```python
from build123d import *

# Parameters (mm, degrees)
SKETCH1_R           = 4
SKETCH1_R_2         = 2.5
BOSS_EXTRUDE1_DEPTH = 9.6
CUT_EXTRUDE1_START  = -3.3
SKETCH2_R           = 2.5
CUT_EXTRUDE1_DEPTH  = 3.3
CUT_EXTRUDE2_DEPTH  = 228.086239125
SKETCH5_R           = 6
CUT_EXTRUDE3_DEPTH  = 5


with BuildPart() as part:
    # Sketch1 → Boss-Extrude1 (new body)
    with BuildSketch(Plane.XY):
        Polygon((221, 0), (5, 0), (0, -5), (0, -15), (5, -20), (221, -20), (226, -15), (226, -5), align=None)
        with Locations((38, -14)):
            Circle(SKETCH1_R, mode=Mode.SUBTRACT)
        with Locations((188, -14)):
            Circle(SKETCH1_R, mode=Mode.SUBTRACT)
        with Locations((16, -10)):
            Circle(SKETCH1_R_2, mode=Mode.SUBTRACT)
        with Locations((60, -10)):
            Circle(SKETCH1_R_2, mode=Mode.SUBTRACT)
        with BuildLine():
            ThreePointArc((98, -8.25), (100.5, -5.75), (103, -8.25))
            Line((103, -8.25), (103, -11.75))
            ThreePointArc((103, -11.75), (100.5, -14.25), (98, -11.75))
            Line((98, -11.75), (98, -8.25))
        make_face(mode=Mode.SUBTRACT)
        with BuildLine():
            Line((128, -8.25), (128, -11.75))
            ThreePointArc((128, -11.75), (125.5, -14.25), (123, -11.75))
            Line((123, -11.75), (123, -8.25))
            ThreePointArc((123, -8.25), (125.5, -5.75), (128, -8.25))
        make_face(mode=Mode.SUBTRACT)
        with Locations((166, -10)):
            Circle(SKETCH1_R_2, mode=Mode.SUBTRACT)
        with Locations((210, -10)):
            Circle(SKETCH1_R_2, mode=Mode.SUBTRACT)
    extrude(amount=BOSS_EXTRUDE1_DEPTH)

    # Sketch2 → Cut-Extrude1 (cut)
    # profile 1 of 2: a face of its own
    with BuildSketch(Plane.XY.offset(9.6).offset(CUT_EXTRUDE1_START)):
        with BuildLine():
            Line((48.392304845, -20), (113, -20))
            Line((113, -20), (113, 0))
            Line((113, 0), (5, 0))
            Line((5, 0), (0, -5))
            Line((0, -5), (0, -15))
            Line((0, -15), (5, -20))
            Line((5, -20), (27.607695155, -20))
            ThreePointArc((27.607695155, -20), (34.894171459, -2.408890085), (50, -14))
            ThreePointArc((50, -14), (49.591109915, -17.105828541), (48.392304845, -20))
        make_face()
        with Locations((16, -10)):
            Circle(SKETCH2_R, mode=Mode.SUBTRACT)
        with Locations((60, -10)):
            Circle(SKETCH2_R, mode=Mode.SUBTRACT)
        with BuildLine():
            Line((98, -11.75), (98, -8.25))
            ThreePointArc((98, -8.25), (100.5, -5.75), (103, -8.25))
            Line((103, -8.25), (103, -11.75))
            ThreePointArc((103, -11.75), (100.5, -14.25), (98, -11.75))
        make_face(mode=Mode.SUBTRACT)
    # profile 2 of 2: a face of its own
    with BuildSketch(Plane.XY.offset(9.6).offset(CUT_EXTRUDE1_START)):
        with BuildLine():
            Line((113, 0), (113, -20))
            Line((113, -20), (177.607695155, -20))
            ThreePointArc((177.607695155, -20), (184.894171459, -2.408890085), (200, -14))
            ThreePointArc((200, -14), (199.591109915, -17.105828541), (198.392304845, -20))
            Line((198.392304845, -20), (221, -20))
            Line((221, -20), (226, -15))
            Line((226, -15), (226, -5))
            Line((226, -5), (221, 0))
            Line((221, 0), (113, 0))
        make_face()
        with BuildLine():
            Line((123, -11.75), (123, -8.25))
            ThreePointArc((123, -8.25), (125.5, -5.75), (128, -8.25))
            Line((128, -8.25), (128, -11.75))
            ThreePointArc((128, -11.75), (125.5, -14.25), (123, -11.75))
        make_face(mode=Mode.SUBTRACT)
        with Locations((166, -10)):
            Circle(SKETCH2_R, mode=Mode.SUBTRACT)
        with Locations((210, -10)):
            Circle(SKETCH2_R, mode=Mode.SUBTRACT)
    extrude(amount=CUT_EXTRUDE1_DEPTH, mode=Mode.SUBTRACT)

    # Sketch4 → Cut-Extrude2 (cut, through all)
    with BuildSketch(Plane.XZ.offset(20)):
        Polygon((149, 4.7), (152, 6.3), (113, 6.3), (74, 6.3), (77, 4.7), (91, 4.7), (91, 1.7), (135, 1.7), (135, 4.7), align=None)
    extrude(amount=-CUT_EXTRUDE2_DEPTH, mode=Mode.SUBTRACT)

    # Sketch5 → Cut-Extrude3 (cut)
    with BuildSketch(Plane.XY.offset(6.3)):
        with Locations((16, -10)):
            Circle(SKETCH5_R)
        with Locations((60, -10)):
            Circle(SKETCH5_R)
        with Locations((166, -10)):
            Circle(SKETCH5_R)
        with Locations((210, -10)):
            Circle(SKETCH5_R)
    extrude(amount=-CUT_EXTRUDE3_DEPTH, mode=Mode.SUBTRACT)


solid = part.part
```
Could you check a few things on this model? Use its own coordinates, in mm. A direction names the side the tool comes from. Coordinates: 2 decimals unless noted, no trailing zeros. Write each loop counter-clockwise with the first axis right and the second up, starting at its lowest first coordinate (ties: lowest second). Pieces come first, ordered by that corner, then holes. Notation, with made-up numbers: (-34.5, 72) -> (11.5, 72) arc R15 ccw to (11.5, 93) -> close; hole circle Ø10 at (-36.75, -36). An arc over 180 degrees is marked (long way). Return JSON: item names as keys, results as strings.
(1) I need wall thicknesses on L1, parallel to X at y = -13.5, z = 8.25; L2, parallel to Y at x = 166, z = 2.7; L3, parallel to Y at x = 38, z = 6.25. Which ranges of each line are inside material? Lowest first, please.
Numbers:
{"L1": "x = 26.01 to 34.03, 41.97 to 49.99, 176.01 to 184.03, 191.97 to 199.99", "L2": "y = -20 to -16, -4 to 0", "L3": "y = -20 to -18, -10 to 0"}
(2) Imagine slicing it at B-B, the plane x = 100.5. Please give me the cut outline in (y, z).
Numbers:
{"outline": "(-20, 0) -> (-14.25, 0) -> (-14.25, 1.7) -> (-20, 1.7) -> close; (-5.75, 0) -> (0, 0) -> (0, 1.7) -> (-5.75, 1.7) -> close"}
(3) I'm going to push flat-ended pins straight in: pin 1 (11 mm diameter, centred on x = 141, y = -5, fed in from +Z); pin 2 (3 mm diameter, centred on y = -17, z = 2.5, fed in from -X); pin 3 (9.5 mm diameter, centred on x = 61.5, y = -10.5, fed in from +Z). Where does each tip first touch, or does it pass through?
Numbers:
{"pin 1": "stops at z = 4.7", "pin 2": "stops at x = 0.5", "pin 3": "stops at z = 6.3"}
(4) Which directions (+Z, -Z, +X, -X, +Y, -Y) give clear straight access to the entire face, cutting with the end or side of a thin tool? Please do faces 4 (the flat face through (84, -10, 4.7)), 5 (the flat face through (185, -11, 9.6)), 6 (the flat face through (166, -13, 1.3)).
Numbers:
{"face 4": "+Z, +Y, -Y", "face 5": "+Z, +X, -X, +Y, -Y", "face 6": "+Z"}
(5) We'd pull the mould along X, two halves only. Please class faces 1 (the flat face through (226, -10, 3)), 2 (the cylindrical face through (212.31, -10.96, 0.64)), 3 (the flat face through (3, -2, 3)): +X half, -X half, draft (parallel to the pull), parting line (faces both ways), or undercut.
Numbers:
{"face 1": "+X half", "face 2": "undercut", "face 3": "-X half"}
(6) Imagine slicing it at A-A, the plane x = 166. Please give me the cut outline in (y, z).
Numbers:
{"outline": "(-20, 0) -> (-12.5, 0) -> (-12.5, 1.3) -> (-16, 1.3) -> (-16, 6.3) -> (-20, 6.3) -> close; (-7.5, 0) -> (0, 0) -> (0, 6.3) -> (-4, 6.3) -> (-4, 1.3) -> (-7.5, 1.3) -> close"}
